The model under review builds one solid part; all positions refer to its coordinate system, in mm. A direction names the side the tool comes from. Give positions to 0.01 mm unless a question says otherwise; leave off trailing zeros. Order: outer loops, then holes, each group sorted by start corner. A loop starts at its lowest first (then second) coordinate and runs counter-clockwise, first axis right, second up. Notation, with made-up numbers: (3, 4) - (26, 4) arc R21 cw to (26, 24) - close; hole circle Ø5 at (-25, 8). An arc over 180 degrees is marked (long way). Answer as CSV lines item,"result". Start each with the question number.
from build123d import *

# Parameters (mm, degrees)
SALIENTE_EXTRUIR1_DEPTH = 4


with BuildPart() as part:
    # Croquis3 → Saliente-Extruir1 (new body)
    with BuildSketch(Plane(origin=(0, 0, 0), x_dir=(1, 0, 0), z_dir=(0, 1, 0))):
        with BuildLine():
            ThreePointArc((402.347998687, -260.746007142), (404.734398392, -259.99334246), (405.982912796, -257.824790071))
            ThreePointArc((405.982912796, -257.824790071), (405.877105548, -257.620612188), (405.7674051, -257.418499365))
            ThreePointArc((405.7674051, -257.418499365), (403.271107475, -257.23416883), (401.314373797, -258.795153423))
            ThreePointArc((401.314373797, -258.795153423), (400.302743654, -257.677442632), (399.088021884, -256.784624632))
            ThreePointArc((399.088021884, -256.784624632), (400.432306585, -254.674101872), (399.9948055, -252.210364776))
            ThreePointArc((399.9948055, -252.210364776), (399.782509433, -252.121967031), (399.568558396, -252.037653715))
            ThreePointArc((399.568558396, -252.037653715), (397.537798087, -253.501037517), (397.042234682, -255.954585253))
            ThreePointArc((397.042234682, -255.954585253), (395.548830385, -255.748632435), (394.044407175, -255.845502269))
            ThreePointArc((394.044407175, -255.845502269), (393.71757112, -253.364658487), (391.798766166, -251.758546653))
            ThreePointArc((391.798766166, -251.758546653), (391.579316968, -251.827291333), (391.36122541, -251.900228661))
            ThreePointArc((391.36122541, -251.900228661), (390.746217737, -254.326593255), (391.943704228, -256.524661881))
            ThreePointArc((391.943704228, -256.524661881), (390.667306245, -257.326834648), (389.577117935, -258.368065845))
            ThreePointArc((389.577117935, -258.368065845), (387.732091346, -256.677715418), (385.229812687, -256.680746422))
            ThreePointArc((385.229812687, -256.680746422), (385.105893077, -256.874467128), (384.985708462, -257.070526914))
            ThreePointArc((384.985708462, -257.070526914), (386.074222349, -259.324549341), (388.404441499, -260.238638117))
            ThreePointArc((388.404441499, -260.238638117), (387.942290632, -261.673590916), (387.776448448, -263.171979827))
            ThreePointArc((387.776448448, -263.171979827), (385.276539772, -263.063056507), (383.361631401, -264.673812109))
            ThreePointArc((383.361631401, -264.673812109), (383.391224742, -264.901864769), (383.425182787, -265.12930846))
            ThreePointArc((383.425182787, -265.12930846), (385.707890489, -266.156306575), (388.080506861, -265.358703205))
            ThreePointArc((388.080506861, -265.358703205), (388.648848637, -266.755005674), (389.484951979, -268.009439474))
            ThreePointArc((389.484951979, -268.009439474), (387.499896269, -269.532909692), (387.068365096, -271.997699444))
            ThreePointArc((387.068365096, -271.997699444), (387.237624334, -272.153375684), (387.409835692, -272.305779849))
            ThreePointArc((387.409835692, -272.305779849), (389.818632906, -271.625209821), (391.123472929, -269.489121785))
            ThreePointArc((391.123472929, -269.489121785), (392.456373915, -270.193428481), (393.903200739, -270.616943654))
            ThreePointArc((393.903200739, -270.616943654), (393.361827622, -273.059958764), (394.615591878, -275.225480148))
            ThreePointArc((394.615591878, -275.225480148), (394.845318735, -275.235937326), (395.075203798, -275.241990362))
            ThreePointArc((395.075203798, -275.241990362), (396.482987537, -273.172298471), (396.109502064, -270.697225101))
            ThreePointArc((396.109502064, -270.697225101), (397.583283074, -270.379983093), (398.963847028, -269.774412182))
            ThreePointArc((398.963847028, -269.774412182), (400.119471003, -271.993858263), (402.471880459, -272.846839757))
            ThreePointArc((402.471880459, -272.846839757), (402.654583186, -272.707184842), (402.834576178, -272.564054467))
            ThreePointArc((402.834576178, -272.564054467), (402.582628784, -270.07367255), (400.705575818, -268.417728184))
            ThreePointArc((400.705575818, -268.417728184), (401.630638339, -267.227378533), (402.298958206, -265.876074898))
            ThreePointArc((402.298958206, -265.876074898), (404.610849972, -266.833448463), (406.961186099, -265.974770545))
            ThreePointArc((406.961186099, -265.974770545), (407.011376059, -265.750349625), (407.057256258, -265.525008131))
            ThreePointArc((407.057256258, -265.525008131), (405.263466718, -263.779213565), (402.761140203, -263.717232975))
            ThreePointArc((402.761140203, -263.717232975), (402.7046372, -262.210753513), (402.347998687, -260.746007142))
        make_face()
        with BuildLine():
            Line((397.264195322, -265.143672214), (393.288016252, -265.143672214))
            ThreePointArc((393.288016252, -265.143672214), (392.526105787, -263.243672214), (393.288016252, -261.343672214))
            Line((393.288016252, -261.343672214), (397.264195322, -261.343672214))
            ThreePointArc((397.264195322, -261.343672214), (398.026105787, -263.243672214), (397.264195322, -265.143672214))
        make_face(mode=Mode.SUBTRACT)
    extrude(amount=SALIENTE_EXTRUIR1_DEPTH)


solid = part.part
Item 1: Machinability: for faces 3 (the face through (395, 0, 261)), 4 (the face through (392.526, 1.972, 263.273)), which of the approach directions +Z, -Z, +X, -X, +Y, -Y give a long, thin tool a straight path to every point of the face, cutting with its end or side? Answer none if there is none.
Item 2: Take a section at D-D on x = 390. Write out the cut boundary in (y, z), and give its area (3 significant figures).
Item 3: Clearance check with flat-ended pins moving along their axes: pin 1 (1 mm diameter, centred on y = 1.5, z = 255.5, fed in from -X); pin 2 (1.5 mm diameter, centred on x = 390.5, y = 3, fed in from +Z); pin 3 (2 mm diameter, centred on y = 1.5, z = 270.5, fed in from +X). State where each tip first meets the part, or that it passes through.
Item 4: Mouldability with a two-part tool opening along X and no side actions: class faces 1 (the face through (395, 4, 261)), 2 (the face through (390.7, 2, 257.3)) as released by +X, released by -X, zero draft, split by the parting line, or undercut.
Item 5: For line 1 along X through (y, z) = (3.2, 266.5); line 2 along Z through (x, y) = (397.5, 1.8); line 3 along Z through (x, y) = (396.25, 1.5), list the stretches that pass through material, from the lowest coordinate up.
Item 6: Take a section at C-C on x = 401. Write out the cut boundary in (y, z), and give its area (3 significant figures).
Item 7: Take a section at A-A on x = 404. Write out the cut boundary in (y, z), and give its area (3 significant figures).
Item 8: Take a section at B-B on z = 271.25. Write out the cut boundary in (x, y).
Data:
1,face 3,"+Z, -Z, +X, -X, -Y"
1,face 4,"+Y, -Y"
2,outline,"(0, 257.91) - (4, 257.91) - (4, 271.48) - (0, 271.48) - close"
2,area,"54.3 mm^2"
3,pin 1,"stops at x = 390.9"
3,pin 2,"stops at z = 271.68"
3,pin 3,"stops at x = 402.96"
4,face 1,"zero draft"
4,face 2,"undercut"
5,line 1,"x = 388.52 to 402.03, 403.2 to 406.16"
5,line 2,"z = 253.56 to 261.63, 264.86 to 270.41"
5,line 3,"z = 255.81 to 261.34, 265.14 to 270.68, 270.97 to 273.85"
6,outline,"(0, 258.4) - (4, 258.4) - (4, 268.09) - (0, 268.09) - close; (0, 268.54) - (4, 268.54) - (4, 272.55) - (0, 272.55) - close"
6,area,"54.8 mm^2"
7,outline,"(0, 257.09) - (4, 257.09) - (4, 260.45) - (0, 260.45) - close; (0, 263.51) - (4, 263.51) - (4, 266.77) - (0, 266.77) - close"
7,area,"26.4 mm^2"
8,outline,"(387, 0) - (390.24, 0) - (390.24, 4) - (387, 4) - close; (393.57, 0) - (396.37, 0) - (396.37, 4) - (393.57, 4) - close; (399.48, 0) - (402.94, 0) - (402.94, 4) - (399.48, 4) - close"
